Autodesk Inventor part; units mm, degrees
ref_plane "YZ Plane" through (0, 0, 0) normal (1, 0, 0) x (0, 1, 0)
ref_plane "XZ Plane" through (0, 0, 0) normal (0, 1, 0) x (-1, 0, 0)
ref_plane "XY Plane" through (0, 0, 0) normal (0, 0, 1) x (1, 0, 0)
sketch "Sketch1" plane through (0, 0, 0) normal (0, 0, 1) x (1, 0, 0)
  circle A0 centre (0, 0) radius 10
  circle A1 centre (0, 0) radius 8.5
  dimension "d0" = 20
  dimension "d1" = 17
extrude "Extrusion1" add sketch "Sketch1" along normal blind 1 contours A0 | A1
sketch "Sketch2" plane through (0, 0, 1) normal (0, 0, 1) x (1, 0, 0)
  circle A0 centre (0, 0) radius 8.5
  dimension "d4" = 17
extrude "Extrusion2" add sketch "Sketch2" along normal blind 2
sketch "Sketch3" plane through (0, 0, 3) normal (0, 0, 1) x (1, 0, 0)
  circle A0 centre (0, 0) radius 10
extrude "Extrusion3" add sketch "Sketch3" along normal blind 1
sketch "Sketch4" plane through (0, 0, 4) normal (0, 0, 1) x (1, 0, 0)
  circle A0 centre (0, 0) radius 4.5
  line L0 (-3.1, 1.51) -> (3.1, 1.51)
  line L1 (3.1, 1.51) -> (3.1, -1.69)
  line L2 (3.1, -1.69) -> (-3.1, -1.69)
  line L3 (-3.1, -1.69) -> (-3.1, 1.51)
  dimension "d9" = 9
  dimension "d10" = 6.2
  dimension "d11" = 3.2
  dimension "d12" = 1.51
  dimension "d13" = 3.1
extrude "Extrusion4" add sketch "Sketch4" along normal blind 7
sketch "Sketch5" plane through (0, 0, 4) normal (0, 0, 1) x (1, 0, 0)
  circle A0 centre (0, 0) radius 8.5
  circle A1 centre (0, 8.5) radius 1
  dimension "d16" = 2
extrude "Extrusion5" cut sketch "Sketch5" against normal blind 7 contours A1 A0 | A0 A1 picked at (0.0387, 8.1646) picked at (0.0312, 8.8275)
properties part number "Stpper Wheel 2"
Source: CAD feature listing. Evaluate the final solid. Frame: model axes, mm. A direction names the side the tool comes from. Round coordinates to 2 decimals unless told otherwise and drop trailing zeros. Write each loop counter-clockwise with the first axis right and the second up, starting at its lowest first coordinate (ties: lowest second). Pieces come first, ordered by that corner, then holes. Notation, with made-up numbers: M 81.5,38.25 L 91.5,38.25 A14 cw 91.5,54.25 Z; hole C 28,58 d8. An arc over 180 degrees is marked long. One line per item, written item: value. Start each with the question number.
Item 1: Mould query, pull axis X, two halves, no side actions, for faces 4 (the flat face through (0, 1.51, 7)), 5 (the cylindrical face through (-0.217, 7.524, 2.028)), 6 (the flat face through (-4.5, -7.4, 1)), 7 (the cylindrical face through (0.36, -8.492, 1.986)). Classes: pulls with the +X half, pulls with the -X half, needs draft (parallel to the pull), parting line crosses it, or undercut.
Item 2: Section query B-B (z = 6). Return the cut outline in (x, y).
Item 3: Pin query (flat end, axial travel): pin 1 (2.5 mm diameter, centred on y = -1, z = 6.5, fed in from +X); pin 2 (1 mm diameter, centred on y = 0.5, z = 6, fed in from -X); pin 3 (3 mm diameter, centred on x = -6.5, y = 5.5, fed in from +Z); pin 4 (1.6 mm diameter, centred on x = 0, y = 8.5, fed in from -Z). Return the tip coordinate at first contact, or that it passes through.
Item 4: Ray query, L1, parallel to Y at x = 0, z = 4.5; L2, parallel to Z at x = -6, y = 6.25; L3, parallel to Z at x = 7.5, y = -2. Return the intervals inside material, ascending. Write a range as from..to.
Item 5: Section query C-C (y = 0). Return the cut outline in (x, z).
Item 6: Set-up query: faces 1 (the cylindrical face through (-2.17, 9.76, 0.49)), 2 (the cylindrical face through (-0.59, -4.46, 7.45)), 3 (the flat face through (-4.5, -7.4, 3)). Return all of +Z, -Z, +X, -X, +Y, -Y with unobstructed straight access to the full face (end or side cutting, diameter ignored); none if empty.
Item 7: Section query D-D (x = -6). Return the cut outline in (y, z).
Item 8: Section query A-A (x = 0). Return the cut outline in (y, z), plus the area to 3 significant figures.
Result set:
1. face 4: undercut
1. face 5: undercut
1. face 6: needs draft
1. face 7: parting line crosses it
2. outline: C 0,0 d9; hole M -3.1,-1.69 L 3.1,-1.69 L 3.1,1.51 L -3.1,1.51 Z
3. pin 1: stops at x = 4.5
3. pin 2: stops at x = -4.5
3. pin 3: stops at z = 4
3. pin 4: passes through
4. L1: y = -4.5..-1.69, 1.51..4.5
4. L2: z = 0..1, 3..4
4. L3: z = 0..4
5. outline: M -10,0 L 10,0 L 10,1 L 8.5,1 L 8.5,3 L 10,3 L 10,4 L 4.5,4 L 4.5,11 L 3.1,11 L 3.1,4 L -3.1,4 L -3.1,11 L -4.5,11 L -4.5,4 L -10,4 L -10,3 L -8.5,3 L -8.5,1 L -10,1 Z
6. face 1: +Z, -Z
6. face 2: +Z
6. face 3: none
7. outline: M -8,0 L 8,0 L 8,1 L 6.02,1 L 6.02,3 L 8,3 L 8,4 L -8,4 L -8,3 L -6.02,3 L -6.02,1 L -8,1 Z
8. outline: M -10,0 L 7.5,0 L 7.5,4 L 4.5,4 L 4.5,11 L 1.51,11 L 1.51,4 L -1.69,4 L -1.69,11 L -4.5,11 L -4.5,4 L -10,4 L -10,3 L -8.5,3 L -8.5,1 L -10,1 Z; M 9.5,0 L 10,0 L 10,1 L 9.5,1 Z; M 9.5,3 L 10,3 L 10,4 L 9.5,4 Z
8. area: 109 mm²
